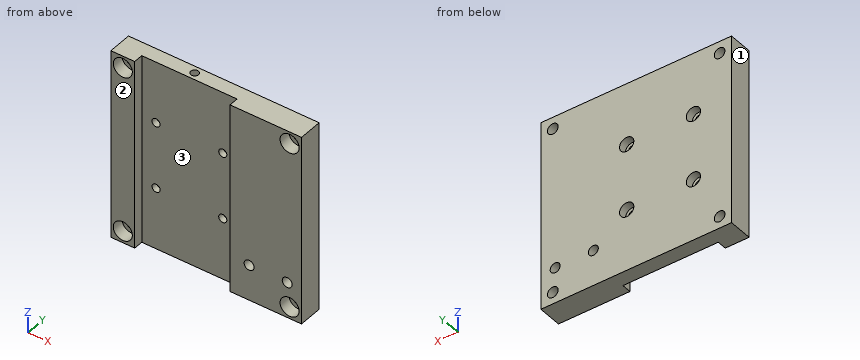
from build123d import *

# Parameters (mm, degrees)
SKETCH_1_W                = 80
SKETCH_1_H                = 80
EXTRUDE_1_DEPTH           = 10
SKETCH_2_W                = 40
SKETCH_2_H                = 4
CUT_EXTRUDE_1_DEPTH       = 91
HOLE_WIZARD_1_D           = 3.4
HOLE_WIZARD_1_CBORE_D     = 6
HOLE_WIZARD_1_CBORE_DEPTH = 3.4
HOLE_WIZARD_M5_1_D        = 4.2
HOLE_WIZARD_2_D           = 4.5
HOLE_WIZARD_2_CBORE_D     = 8
HOLE_WIZARD_2_CBORE_DEPTH = 5
HOLE_WIZARD_M4_1_D        = 3.3
HOLE_WIZARD_M4_1_DEPTH    = 10.1
HOLE_WIZARD_M4_1_TIP      = 0.991420021


with BuildPart() as part:
    # 草图1 → 凸台-拉伸1 (new body)
    with BuildSketch(Plane(origin=(0, 0, 0), x_dir=(1, 0, 0), z_dir=(0, 1, 0))):
        Rectangle(SKETCH_1_W, SKETCH_1_H)
    extrude(amount=EXTRUDE_1_DEPTH)

    # 草图2 → 切除-拉伸1 (cut, through all)
    with BuildSketch(Plane.XY.offset(40)):
        with Locations((-10, 2)):
            Rectangle(SKETCH_2_W, SKETCH_2_H)
    extrude(amount=-CUT_EXTRUDE_1_DEPTH, mode=Mode.SUBTRACT)

    # 打孔尺寸根据内六角圆柱头螺钉的类型1 (through all)
    with Locations(Plane(origin=(0, 10, 0), x_dir=(1, 0, 0), z_dir=(0, 1, 0))):
        with Locations((-24, 14), (4, 14), (4, -14), (-24, -14)):
            CounterBoreHole(HOLE_WIZARD_1_D / 2, HOLE_WIZARD_1_CBORE_D / 2, HOLE_WIZARD_1_CBORE_DEPTH)

    # M5 螺纹孔1 (through all)
    with Locations(Plane(origin=(0, 0, 0), x_dir=(-1, 0, 0), z_dir=(0, -1, 0))):
        with Locations((-18, 25), (-34, 25)):
            Hole(HOLE_WIZARD_M5_1_D / 2)

    # 打孔尺寸根据内六角圆柱头螺钉的类型2 (through all)
    with Locations(Plane(origin=(0, 0, 0), x_dir=(-1, 0, 0), z_dir=(0, -1, 0))):
        with Locations((35, -35), (-35, -35), (-35, 35), (35, 35)):
            CounterBoreHole(HOLE_WIZARD_2_D / 2, HOLE_WIZARD_2_CBORE_D / 2, HOLE_WIZARD_2_CBORE_DEPTH)

    # M4 螺纹孔1
    with Locations(Plane.XY.offset(40)):
        with Locations((-10, 7)):
            Hole(HOLE_WIZARD_M4_1_D / 2, depth=HOLE_WIZARD_M4_1_DEPTH)
            with Locations((0, 0, -(HOLE_WIZARD_M4_1_DEPTH + HOLE_WIZARD_M4_1_TIP / 2))):  # 118° drill point
                Cone(0, HOLE_WIZARD_M4_1_D / 2, HOLE_WIZARD_M4_1_TIP, mode=Mode.SUBTRACT)


solid = part.part
CAD build for the part. Positions are in the model's coordinates, mm. Face numbers are marked on the shaded views. Coordinates: 2 decimals unless noted, no trailing zeros. Loops run counter-clockwise (first coordinate to the right, second up) from the corner with the lowest first, then second, coordinate; pieces in that order, holes last. Notation, with made-up numbers: (47, 11) - (56, 11) arc R18 ccw to (56, 33) - close; hole circle Ø2 at (89, 4.5). An arc over 180 degrees is marked (long way). Write item = value, one per line. Start each with the question number.
Q1. Drill centre lines: L1, parallel to X at y = 1.55, z = -35; L2, parallel to Z at x = -35, y = 7.45. Where is each one in solid material? Low to high.
Q2. Cut at B-B, the plane y = 1. List the corners of the cut face in (x, z).
Q3. Pull direction X, two halves, no side cores. Call the marked faces 1, 2 and 3: pulls with the +X half, pulls with the -X half, needs draft (parallel to the pull), parting line crosses it, or undercut.
Q4. Cut at C-C, the plane x = -35. List the corners of the cut face in (y, z), then the cut area to 3 significant figures.
Q5. Cut at D-D, the plane z = -35. List the corners of the cut face in (x, y), then the cut area to 3 significant figures.
Q6. Cut at A-A, the plane z = 35. List the corners of the cut face in (x, y), then the cut area to 3 significant figures.
Q7. Flat gauge pins, fed straight in: pin 1 Ø2.5 at (x, z) = (35, 35) entering from -Y; pin 2 Ø5.5 at (x, z) = (-24, -14) entering from +Y; pin 3 Ø2.5 at (x, z) = (-33.5, -37) entering from -Y; pin 4 Ø3.5 at (x, z) = (-24, 14) entering from -Y. Where does each tip first touch, or does it go through?
Computed:
q1.L1 = -40 to -39, -31 to -30, 10 to 31, 39 to 40
q1.L2 = -40 to -37.25, -32.75 to 32.75, 37.25 to 40
q2.outline = (-40, -40) - (-30, -40) - (-30, 40) - (-40, 40) - close; (10, -40) - (40, -40) - (40, 40) - (10, 40) - close; hole circle Ø8 at (-35, -35); hole circle Ø8 at (-35, 35); hole circle Ø4.2 at (18, -25); hole circle Ø8 at (35, -35); hole circle Ø8 at (35, 35); hole circle Ø4.2 at (34, -25)
q3.face_1 = pulls with the -X half
q3.face_2 = needs draft
q3.face_3 = undercut
q4.outline = (0, -40) - (10, -40) - (10, -37.25) - (5, -37.25) - (5, -39) - (0, -39) - close; (0, -31) - (5, -31) - (5, -32.75) - (10, -32.75) - (10, 32.75) - (5, 32.75) - (5, 31) - (0, 31) - close; (0, 39) - (5, 39) - (5, 37.25) - (10, 37.25) - (10, 40) - (0, 40) - close
q4.area = 675 mm²
q5.outline = (-40, 0) - (-39, 0) - (-39, 5) - (-37.25, 5) - (-37.25, 10) - (-40, 10) - close; (-32.75, 5) - (-31, 5) - (-31, 0) - (-30, 0) - (-30, 4) - (10, 4) - (10, 0) - (31, 0) - (31, 5) - (32.75, 5) - (32.75, 10) - (-32.75, 10) - close; (37.25, 5) - (39, 5) - (39, 0) - (40, 0) - (40, 10) - (37.25, 10) - close
q5.area = 515 mm²
q6.outline = (-40, 0) - (-39, 0) - (-39, 5) - (-37.25, 5) - (-37.25, 10) - (-40, 10) - close; (-32.75, 5) - (-31, 5) - (-31, 0) - (-30, 0) - (-30, 4) - (10, 4) - (10, 0) - (31, 0) - (31, 5) - (32.75, 5) - (32.75, 10) - (-32.75, 10) - close; (37.25, 5) - (39, 5) - (39, 0) - (40, 0) - (40, 10) - (37.25, 10) - close; hole circle Ø3.3 at (-10, 7)
q6.area = 506 mm²
q7.pin_1 = through
q7.pin_2 = 6.6
q7.pin_3 = 5
q7.pin_4 = 4
